Solid Edge part; units mm, degrees
sketch "Sketch1" plane through (0, 0, 0) normal (0, 0, 1) x (1, 0, 0)
  circle A0 centre (0, 0) radius 10
extrude "Protrusion1" add sketch "Sketch1" along normal blind 5.5
sketch "Sketch2" plane through (0, 0, 0) normal (0, 0, -1) x (1, 0, 0)
  circle A0 centre (0, 0) radius 5
extrude "Protrusion2" add sketch "Sketch2" along normal blind 29.5
sketch "Sketch3" plane through (0, 0, -29.5) normal (0, 0, -1) x (1, 0, 0)
  circle A0 centre (0, 0) radius 4.9997
extrude "Cutout1" cut sketch "Sketch3" against normal blind 26 flip side to cut
chamfer "Chamfer_1" distance 0.75 angle 45 1 edges at (-4.9997, 0, -29.5)
sketch "Sketch4" plane through (0, 0, 5.5) normal (0, 0, 1) x (1, 0, 0)
  line L0 (-1.7321, 3) -> (1.7321, 3)
  line L1 (3.4641, 0) -> (1.7321, 3)
  line L2 (1.7321, -3) -> (3.4641, 0)
  line L3 (-1.7321, -3) -> (1.7321, -3)
  line L4 (-3.4641, 0) -> (-1.7321, -3)
  line L5 (-1.7321, 3) -> (-3.4641, 0)
extrude "Cutout2" cut sketch "Sketch4" against normal blind 3.6667
sketch "Sketch5" plane through (0, 0, 0) normal (0, -1, 0) x (1, 0, 0)
  line L0 (10, 5.5) -> (4.5, 0)
  line L1 (4.5, 0) -> (10, 0)
  line L2 (10, 0) -> (10, 5.5)
revolve "RevolvedCutout1" cut sketch "Sketch5" angle 360 about axis through (0, 0, 14.0017) along (0, 0, -1)
properties part number "185738" material "Stainless Steel, 304"
Check sheet for the modelled part. Datum: model origin and axes. Units: mm. A direction names the side the tool comes from. Round coordinates to 2 decimals unless told otherwise and drop trailing zeros. Order: outer loops, then holes, each group sorted by start corner. A loop starts at its lowest first (then second) coordinate and runs counter-clockwise, first axis right, second up. Notation, with made-up numbers: (67.5, 46.25) -> (87.5, 46.25) arc R19 ccw to (87.5, 52.25) -> close; hole circle Ø9 at (21, 33.5). An arc over 180 degrees is marked (long way). One line per item, written item: value. Start each with the question number.
Q1. Mould release check, pull along Y, two halves, no side actions. Record for faces 1 (the face through (0, 0, -29.5)), 2 (the face through (0, 3, 4)), 3 (the face through (-1.08, -4.88, -1.73)): pulls with the +Y half, pulls with the -Y half, needs draft (parallel to the pull), parting line crosses it, or undercut.
Q2. Cross-section at A-A (z = 3). Record the boundary of the cut face in (x, y), and give its area (3 significant figures).
Q3. Cross-section at C-C (z = -2). Record the boundary of the cut face in (x, y).
Q4. Set-up check for faces 4 (the face through (-2.4, 2.4, 5.5)), 5 (the face through (4.77, -1.5, -16.3)), 6 (the face through (-2.6, 1.5, 3.7)): record each of +Z, -Z, +X, -X, +Y, -Y from which the full face is reachable in a straight line by a thin tool's end or side.
Q5. Gauge pin test, flat ends, axial feed: pin 1 Ø3 at (x, y) = (0.5, -1) entering from +Z; pin 2 Ø1 at (x, z) = (1, 3.5) entering from +Y; pin 3 Ø8 at (x, z) = (2.5, -23) entering from -Y. Record the tip position at first contact, or that the pin passes through.
Q6. Thickness scan on line 1 (Z direction, x = -1.75, y = -1); line 2 (Z direction, x = 1, y = -6); line 3 (Y direction, x = -3.5, z = -12.5). Record the ranges inside material, lowest first.
Completed:
1. face 1: needs draft
1. face 2: undercut
1. face 3: parting line crosses it
2. outline: circle Ø15 at (0, 0); hole (-3.46, 0) -> (-1.73, -3) -> (1.73, -3) -> (3.46, 0) -> (1.73, 3) -> (-1.73, 3) -> close
2. area: 146 mm²
3. outline: circle Ø10 at (0, 0)
4. face 4: +Z, +X, -X, +Y, -Y
4. face 5: -Z
4. face 6: +Z
5. pin 1: stops at z = 1.83
5. pin 2: stops at y = 8.44
5. pin 3: stops at y = -5
6. line 1: z = -29.5 to 1.83
6. line 2: z = 1.58 to 5.5
6. line 3: y = -3.57 to 3.57
